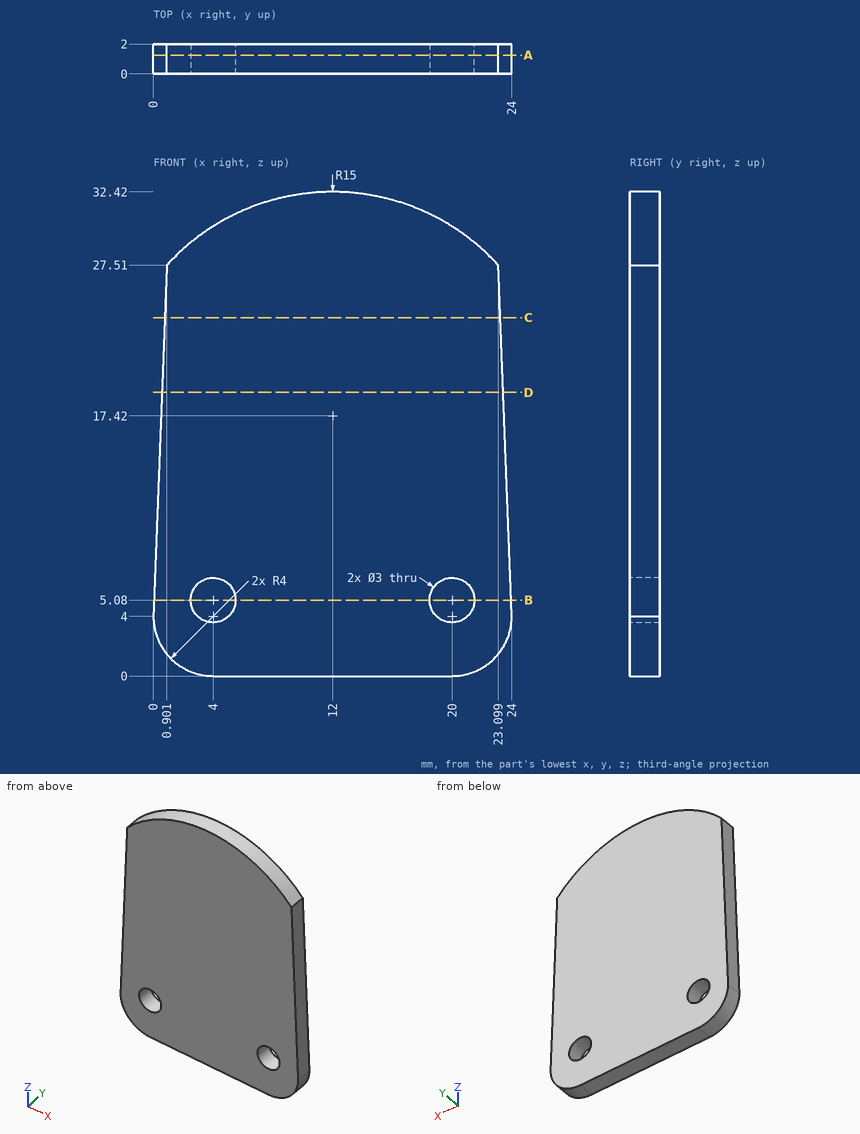
The figure shows three views and two pictorial views of one solid part (mm, origin at its lowest corner). Answer the questions. Give positions to 0.01 mm unless a question says otherwise; leave off trailing zeros. Write each loop counter-clockwise with the first axis right and the second up, starting at its lowest first coordinate (ties: lowest second). Pieces come first, ordered by that corner, then holes. Notation, with made-up numbers: (76, -28) - (128, -28) arc R24 ccw to (128, -9) - close; hole circle Ø11 at (64.25, 58). An arc over 180 degrees is marked (long way). Return JSON: item names as keys, results as strings.
Q1. A cutting plane is placed at D-D, the plane z = 19. Determine the outline of the cut face in (x, y) (1 decimal), and give its area (3 significant figures).
Reply:
{"outline": "(0.6, 0) - (23.4, 0) - (23.4, 2) - (0.6, 2) - close", "area": "45.7 mm²"}
Q2. A cutting plane is placed at A-A, the plane y = 1.25. Determine the outline of the cut face in (x, z).
Reply:
{"outline": "(0, 4) arc R4 ccw to (4, 0) - (20, 0) arc R4 ccw to (24, 4) - (23.1, 27.51) arc R15 ccw to (0.9, 27.51) - close; hole circle Ø3 at (4, 5.08); hole circle Ø3 at (20, 5.08)"}
Q3. Consider line 1 along Z through (x, y) = (4, 1.2); line 2 along Z through (x, y) = (20.5, 0.2) (1 decimal); line 3 along Z through (x, y) = (21.75, 0.5). Determine where each line is inside the solid, lowest interval first. Write a range as [from, to].
Reply:
{"line 1": "[0, 3.58], [6.58, 30.11]", "line 2": "[0, 3.7], [6.5, 29.8]", "line 3": "[0.4, 28.82]"}
Q4. Given P1, Ø2.5, axis at x = 4, z = 5.08, coming from the +Y side, flat-ended and moving along its own axis, determine where the tip first touches the part or whether it passes through.
Reply:
{"P1": "through"}
Q5. A cutting plane is placed at B-B, the plane z = 5.08. Determine the outline of the cut face in (x, y).
Reply:
{"outline": "(0.04, 0) - (2.5, 0) - (2.5, 2) - (0.04, 2) - close; (5.5, 0) - (18.5, 0) - (18.5, 2) - (5.5, 2) - close; (21.5, 0) - (23.96, 0) - (23.96, 2) - (21.5, 2) - close"}
Q6. A cutting plane is placed at C-C, the plane z = 24. Determine the outline of the cut face in (x, y).
Reply:
{"outline": "(0.77, 0) - (23.23, 0) - (23.23, 2) - (0.77, 2) - close"}
